The listing builds one solid part. Answer for the finished solid, in the listing's coordinates (mm). Face numbers are marked on the shaded views. A direction names the side the tool comes from. Give positions to 0.01 mm unless a question says otherwise; leave off trailing zeros. Order: outer loops, then holes, each group sorted by start corner. A loop starts at its lowest first (then second) coordinate and runs counter-clockwise, first axis right, second up. Notation, with made-up numbers: (68, 10.5) - (102, 10.5) arc R19 cw to (102, 39.5) - close; hole circle Ø3 at (5.25, -0.5). An arc over 180 degrees is marked (long way). Answer in a Markdown table with one row per item.
Autodesk Inventor part; units mm, degrees
ref_plane "YZ Plane" through (0, 0, 0) normal (1, 0, 0) x (0, 1, 0)
ref_plane "XZ Plane" through (0, 0, 0) normal (0, 1, 0) x (-1, 0, 0)
ref_plane "XY Plane" through (0, 0, 0) normal (0, 0, 1) x (1, 0, 0)
sketch "Sketch1" plane through (0, 0, 0) normal (0, 0, 1) x (1, 0, 0)
  circle A0 centre (0, 0) radius 3.175
  circle A1 centre (0, 0) radius 2.975
  arc A2 (-4.0862, -4.8606) -> (4.0862, 4.8606) centre (0, 0) ccw
  point P0 (0, 0)
  dimension "d0" = 0.2
extrude "Extrusion1" add sketch "Sketch1" against normal blind 6 contours A1
sketch "Sketch2" plane through (0, 0, 0) normal (0, 0, 1) x (1, 0, 0)
  circle A0 centre (0, 0) radius 2.975
  point P0 (0, 0)
extrude "Extrusion2" add sketch "Sketch2" along normal blind 0.2
sketch "Sketch3" plane through (0, 0, 0.2) normal (0, 0, 1) x (1, 0, 0)
  circle A0 centre (0, 0) radius 6.75
  circle A1 centre (0, 0) radius 19.05
  circle A2 centre (0, 0) radius 8.75
  point P0 (0, 0)
  dimension "d5" = 2
extrude "Extrusion3" add sketch "Sketch3" along normal blind 1 contours A0 | A2
properties part number "CartWheelCap"
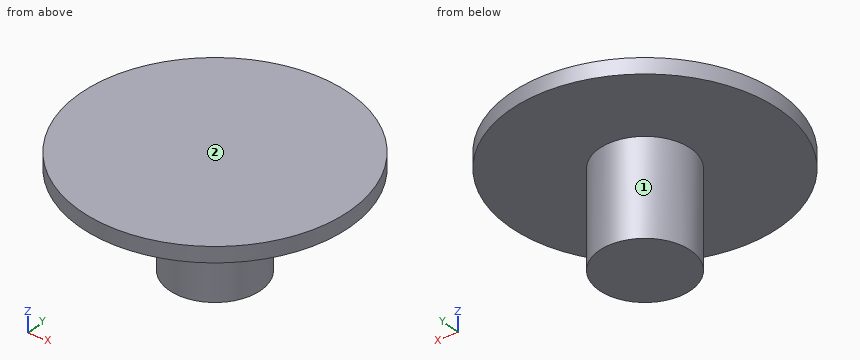
Item 1: Find section D-D on x = -4.75. Write down the section's boundary in (y, z), then the cut area to 3 significant figures.
Answer block:
| item | result |
|---|---|
| outline | (-7.35, 0.2) - (7.35, 0.2) - (7.35, 1.2) - (-7.35, 1.2) - close |
| area | 14.7 mm² |
Item 2: Each of these flat-tipped pins is pushed along its axis until it touches: P1, Ø2, axis at y = 4, z = 0, coming from the +X side; P2, Ø1.5, axis at y = 0.5, z = -3, coming from the -X side (3 decimals). Where does it stop, or does it pass through?
Answer block:
| item | result |
|---|---|
| P1 | x = 8.21 |
| P2 | x = -2.975 |
Item 3: Find section C-C on z = 0.5. Write down the section's boundary in (x, y).
Answer block:
| item | result |
|---|---|
| outline | circle Ø17.5 at (0, 0) |
Item 4: Find section A-A on y = 0. Write down the section's boundary in (x, z) (3 decimals).
Answer block:
| item | result |
|---|---|
| outline | (-8.75, 0.2) - (-2.975, 0.2) - (-2.975, -6) - (2.975, -6) - (2.975, 0.2) - (8.75, 0.2) - (8.75, 1.2) - (-8.75, 1.2) - close |
Item 5: Consider line 1 (Z direction, x = 1.5, y = -5); line 2 (X direction, y = 2.25, z = -2); line 3 (X direction, y = 8, z = 0.5). Determine where each line is inside the solid, lowest interval first.
Answer block:
| item | result |
|---|---|
| line 1 | 0.2 to 1.2 |
| line 2 | -1.95 to 1.95 |
| line 3 | -3.54 to 3.54 |
Item 6: Which of the six approach directions +Z, -Z, +X, -X, +Y, -Y give full straight-line access (tool end or side, diameter ignored) to the marked faces 1 and 2?
Answer block:
| item | result |
|---|---|
| face 1 | -Z |
| face 2 | +Z, +X, -X, +Y, -Y |
